Input: dimensioned drawing with shaded views. Units: mm. Origin: part minimum x, y, z. Round coordinates to 2 decimals unless told otherwise and drop trailing zeros. Order: outer loops, then holes, each group sorted by start corner. A loop starts at its lowest first (then second) coordinate and runs counter-clockwise, first axis right, second up. Notation, with made-up numbers: (86, 67) - (112, 67) arc R15 ccw to (112, 82) - close; hole circle Ø7 at (-32, 4.5). An arc over 180 degrees is marked (long way). Put each result on its own line as item: value. Start each with the question number.
(1) Pin query (flat end, axial travel): P1, Ø3, axis at x = 50, z = 9, coming from the -Y side. Return the tip coordinate at first contact, or that it passes through.
(2) Section B-B (z = 20.5). Output: boundary loops of the cut face in (x, y).
(3) Section A-A (x = 40). Output: boundary loops of the cut face in (y, z).
(4) Section C-C (y = 12.25). Output: boundary loops of the cut face in (x, z).
(5) Pull-direction query (X, two-part tool) for the marked faces 1, 2 and 3; classes: released by +X, released by -X, zero draft, split by the parting line, or undercut.
(6) Material intervals for L1, parallel to Z at x = 40, y = 15; L2, parallel to X at y = 3.75, z = 41; L3, parallel to Z at x = 48.5, y = 13.75, sorted ascending. Write a range as [from, to].
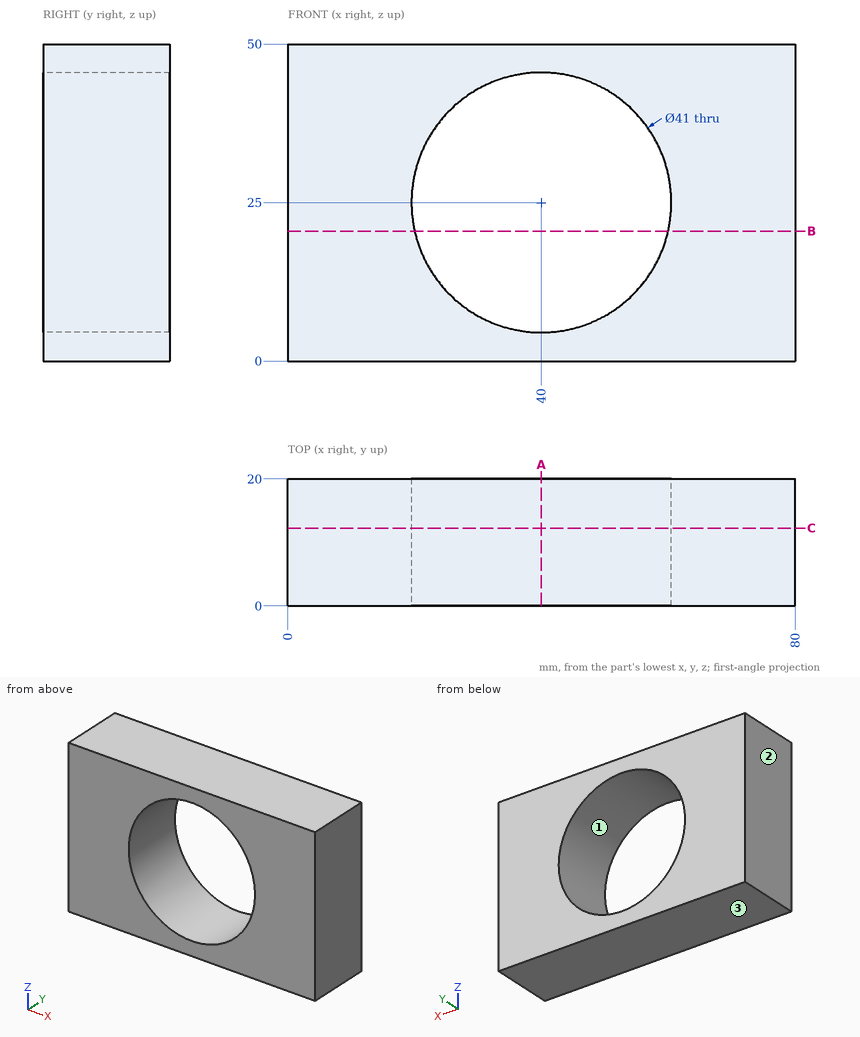
Checks:
1. P1: passes through
2. outline: (0, 0) - (20, 0) - (20, 20) - (0, 20) - close; (60, 0) - (80, 0) - (80, 20) - (60, 20) - close
3. outline: (0, 0) - (20, 0) - (20, 4.5) - (0, 4.5) - close; (0, 45.5) - (20, 45.5) - (20, 50) - (0, 50) - close
4. outline: (0, 0) - (80, 0) - (80, 50) - (0, 50) - close; hole circle Ø41 at (40, 25)
5. face 1: undercut
5. face 2: released by -X
5. face 3: zero draft
6. L1: z = [0, 4.5], [45.5, 50]
6. L2: x = [0, 27.18], [52.82, 80]
6. L3: z = [0, 6.35], [43.65, 50]
